Can you work these out from the drawing? Everything is in mm from the part's minimum corner. Coordinates: 2 decimals unless noted, no trailing zeros. Loops run counter-clockwise (first coordinate to the right, second up) from the corner with the lowest first, then second, coordinate; pieces in that order, holes last.
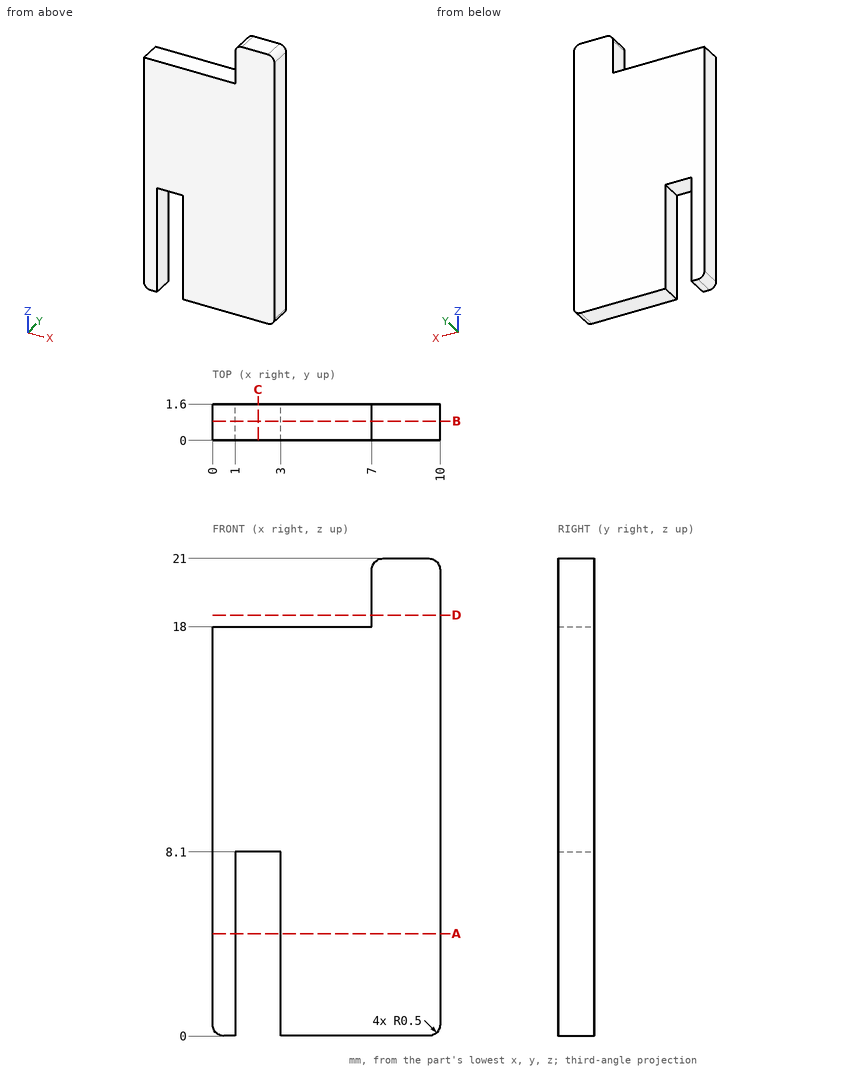
Item 1: Suppose I cut it at A-A, the plane z = 4.5. Please give me the cut outline in (x, y).
Results are:
outline: (0, 0) - (1, 0) - (1, 1.6) - (0, 1.6) - close; (3, 0) - (10, 0) - (10, 1.6) - (3, 1.6) - close
Item 2: Suppose I cut it at B-B, the plane y = 0.85. Please give me the cut outline in (x, z).
Results are:
outline: (0, 0.5) arc R0.5 ccw to (0.5, 0) - (1, 0) - (1, 8.1) - (3, 8.1) - (3, 0) - (9.5, 0) arc R0.5 ccw to (10, 0.5) - (10, 20.5) arc R0.5 ccw to (9.5, 21) - (7.5, 21) arc R0.5 ccw to (7, 20.5) - (7, 18) - (0, 18) - close
Item 3: I'm going to push a flat-ended pin straight in: P1, Ø0.8, axis at x = 2.5, y = 1, coming from the -Z side. Where does the tip first touch, or does it pass through?
Results are:
P1: stops at z = 8.1
Item 4: Suppose I cut it at C-C, the plane x = 2. Please give me the cut outline in (y, z), plus the area to 3 significant figures.
Results are:
outline: (0, 8.1) - (1.6, 8.1) - (1.6, 18) - (0, 18) - close
area: 15.8 mm2
Item 5: I need wall thicknesses on line 1 along X through (y, z) = (0.4, 5.75); line 2 along X through (y, z) = (0.1, 20.25); line 3 along Z through (x, y) = (3.5, 0.45). Which ranges of each line are inside material? Lowest first, please.
Results are:
line 1: x = 0 to 1, 3 to 10
line 2: x = 7 to 10
line 3: z = 0 to 18
Item 6: Suppose I cut it at D-D, the plane z = 18.5. Please give me the cut outline in (x, y), plus the area to 3 significant figures.
Results are:
outline: (7, 0) - (10, 0) - (10, 1.6) - (7, 1.6) - close
area: 4.80 mm2
